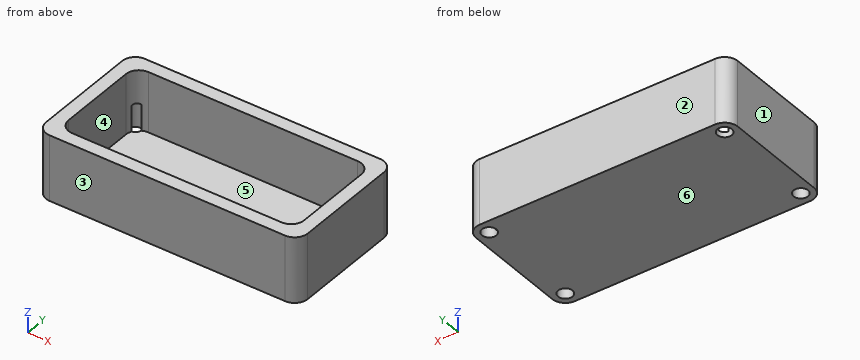
from build123d import *

# Parameters (mm, degrees)
F0_W     = 100
F0_H     = 50
F1_DEPTH = 25
F2_DEPTH = 2
F3_R     = 5
F4_D     = 5.5
F4_DEPTH = 12
F4_TIP   = 1.6523667023


with BuildPart() as f1:
    # F0 (on Top) → F1 (new body)
    with BuildSketch(Plane.XY):
        with Locations((6.475339179, -8.8739781123)):
            Rectangle(F0_W, F0_H)
        with BuildLine():
            ThreePointArc((-38.524660821, 6.1260218877), (-37.0601947269, 9.6615557936), (-33.524660821, 11.1260218877))
            Line((-33.524660821, 11.1260218877), (46.475339179, 11.1260218877))
            ThreePointArc((46.475339179, 11.1260218877), (50.010873085, 9.6615557936), (51.475339179, 6.1260218877))
            Line((51.475339179, 6.1260218877), (51.475339179, -23.8739781123))
            ThreePointArc((51.475339179, -23.8739781123), (50.010873085, -27.4095120182), (46.475339179, -28.8739781123))
            Line((46.475339179, -28.8739781123), (-33.524660821, -28.8739781123))
            ThreePointArc((-33.524660821, -28.8739781123), (-37.0601947269, -27.4095120182), (-38.524660821, -23.8739781123))
            Line((-38.524660821, -23.8739781123), (-38.524660821, 6.1260218877))
        make_face(mode=Mode.SUBTRACT)
    extrude(amount=F1_DEPTH)

    # F0 (on Top) → F2 (join)
    with BuildSketch(Plane.XY):
        with Locations((6.475339179, -8.8739781123)):
            Rectangle(F0_W, F0_H)
        with BuildLine():
            ThreePointArc((-38.524660821, 6.1260218877), (-37.0601947269, 9.6615557936), (-33.524660821, 11.1260218877))
            Line((-33.524660821, 11.1260218877), (46.475339179, 11.1260218877))
            ThreePointArc((46.475339179, 11.1260218877), (50.010873085, 9.6615557936), (51.475339179, 6.1260218877))
            Line((51.475339179, 6.1260218877), (51.475339179, -23.8739781123))
            ThreePointArc((51.475339179, -23.8739781123), (50.010873085, -27.4095120182), (46.475339179, -28.8739781123))
            Line((46.475339179, -28.8739781123), (-33.524660821, -28.8739781123))
            ThreePointArc((-33.524660821, -28.8739781123), (-37.0601947269, -27.4095120182), (-38.524660821, -23.8739781123))
            Line((-38.524660821, -23.8739781123), (-38.524660821, 6.1260218877))
        make_face(mode=Mode.SUBTRACT)
        with BuildLine():
            Line((46.475339179, 11.1260218877), (-33.524660821, 11.1260218877))
            ThreePointArc((-33.524660821, 11.1260218877), (-37.0601947269, 9.6615557936), (-38.524660821, 6.1260218877))
            Line((-38.524660821, 6.1260218877), (-38.524660821, -23.8739781123))
            ThreePointArc((-38.524660821, -23.8739781123), (-37.0601947269, -27.4095120182), (-33.524660821, -28.8739781123))
            Line((-33.524660821, -28.8739781123), (46.475339179, -28.8739781123))
            ThreePointArc((46.475339179, -28.8739781123), (50.010873085, -27.4095120182), (51.475339179, -23.8739781123))
            Line((51.475339179, -23.8739781123), (51.475339179, 6.1260218877))
            ThreePointArc((51.475339179, 6.1260218877), (50.010873085, 9.6615557936), (46.475339179, 11.1260218877))
        make_face()
    extrude(amount=F2_DEPTH)

    # F3
    f3_edges = [f1.edges().sort_by_distance(p)[0] for p in [
        (-43.524661, -33.873978, 12.5),
        (56.475339, -33.873978, 12.5),
        (56.475339, 16.126022, 12.5),
        (-43.524661, 16.126022, 12.5),
    ]]
    fillet(f3_edges, radius=F3_R)

    # F4
    with Locations(Plane(origin=(0, 0, 0), x_dir=(1, 0, 0), z_dir=(0, 0, -1))):
        with Locations((51.475339179, -11.1260218877), (51.475339179, 28.8739781123), (-38.524660821, 28.8739781123), (-38.524660821, -11.1260218877)):
            Hole(F4_D / 2, depth=F4_DEPTH)
            with Locations((0, 0, -(F4_DEPTH + F4_TIP / 2))):  # 118° drill point
                Cone(0, F4_D / 2, F4_TIP, mode=Mode.SUBTRACT)


solid = f1.part
Verification items for the finished model (mm, model axes). Face numbers are marked on the shaded views. A direction names the side the tool comes from. Coordinates: 2 decimals unless noted, no trailing zeros. Loops run counter-clockwise (first coordinate to the right, second up) from the corner with the lowest first, then second, coordinate; pieces in that order, holes last. Notation, with made-up numbers: M 16.5,-21.75 L 55.5,-21.75 A32 cw 55.5,16.25 Z; hole C 5.5,-34 d5. An arc over 180 degrees is marked long. One line per item, written item: value.
1. Section check A-A on z = 18.25. Record the cut outline in (x, y).
Answers follow:
outline: M -43.52,-28.87 A5 ccw -38.52,-33.87 L 51.48,-33.87 A5 ccw 56.48,-28.87 L 56.48,11.13 A5 ccw 51.48,16.13 L -38.52,16.13 A5 ccw -43.52,11.13 Z; hole M -38.52,-23.87 A5 ccw -33.52,-28.87 L 46.48,-28.87 A5 ccw 51.48,-23.87 L 51.48,6.13 A5 ccw 46.48,11.13 L -33.52,11.13 A5 ccw -38.52,6.13 Z
2. Mould release check, pull along Y, two halves, no side actions. Record for the marked faces 1, 2, 3 and 4: pulls with the +Y half, pulls with the -Y half, needs draft (parallel to the pull), parting line crosses it, or undercut.
Answers follow:
face 1: needs draft
face 2: pulls with the +Y half
face 3: pulls with the -Y half
face 4: undercut
3. Material ranges on line 1 along Y through (x, z) = (-17, 14.75); line 2 along X through (y, z) = (-24, 19); line 3 along Z through (x, y) = (34.5, -1.5), recorded low to high. Write a range as from..to.
Answers follow:
line 1: -33.87..-28.87, 11.13..16.13
line 2: -43.52..-38.52, 51.47..56.48
line 3: 0..2
4. Section check B-B on y = -5.5. Record the cut outline in (x, z).
Answers follow:
outline: M -43.52,0 L 56.48,0 L 56.48,25 L 51.48,25 L 51.48,2 L -38.52,2 L -38.52,25 L -43.52,25 Z
5. Section check D-D on z = 6.75. Record the cut outline in (x, y), plus the area to 3 significant figures.
Answers follow:
outline: M -43.52,-28.87 A5 ccw -38.52,-33.87 L 51.48,-33.87 A5 ccw 56.48,-28.87 L 56.48,11.13 A5 ccw 51.48,16.13 L -38.52,16.13 A5 ccw -43.52,11.13 Z; hole M -38.52,-23.87 A5 ccw -37.96,-26.18 A2.75 ccw long -35.83,-28.31 A5 ccw -33.52,-28.87 L 46.48,-28.87 A5 ccw 48.78,-28.31 A2.75 ccw long 50.91,-26.18 A5 ccw 51.48,-23.87 L 51.48,6.13 A5 ccw 50.91,8.43 A2.75 ccw long 48.78,10.56 A5 ccw 46.48,11.13 L -33.52,11.13 A5 ccw -35.83,10.56 A2.75 ccw long -37.96,8.43 A5 ccw -38.52,6.13 Z
area: 1,310 mm^2
6. Gauge pin test, flat end, axial feed: P1, Ø5, axis at x = -38.52, y = -28.87, coming from the -Z side. Record the tip position at first contact, or that the pin passes through.
Answers follow:
P1: z = 12.15
7. Section check C-C on x = -17. Record the cut outline in (y, z), plus the area to 3 significant figures.
Answers follow:
outline: M -33.87,0 L 16.13,0 L 16.13,25 L 11.13,25 L 11.13,2 L -28.87,2 L -28.87,25 L -33.87,25 Z
area: 330 mm^2
8. Set-up check for the marked faces 5 and 6: record each of +Z, -Z, +X, -X, +Y, -Y from which the full face is reachable in a straight line by a thin tool's end or side.
Answers follow:
face 5: +Z
face 6: -Z, +X, -X, +Y, -Y
